Read the model definition and answer for the solid it produces. Units are mm, in the model's axes. A direction names the side the tool comes from. Round coordinates to 2 decimals unless told otherwise and drop trailing zeros. Write each loop counter-clockwise with the first axis right and the second up, starting at its lowest first coordinate (ties: lowest second). Pieces come first, ordered by that corner, then holes. Notation, with made-up numbers: (59.5, -1) -> (112.5, -1) arc R17 ccw to (112.5, 31) -> close; hole circle Ø9 at (67.5, 9). An arc over 180 degrees is marked (long way). Return JSON: item names as keys, results as strings. Group by question number.
(1) The mould has two halves that part along Y. Classify faces 4 (the cylindrical face through (9.127, 29.349, 1.972)), 5 (the cylindrical face through (-0.195, 37.437, 1.972)), 6 (the cylindrical face through (1.014, 38.773, 1.972)): released by +Y, released by -Y, zero draft, split by the parting line, or undercut.
(2) A cutting plane is placed at A-A on y = 25.5. Give the vertices of the cut face in (x, z), then the cut area to 3 significant figures.
(3) Given pin 1 (1.5 mm diameter, centred on x = -10.5, z = 3.5, fed in from -Y); pin 2 (1.5 mm diameter, centred on y = 34.5, z = 1, fed in from +X) (3 decimals), each flat-ended and moving along its own axis, determine where each tip first touches the part or whether it passes through.
(4) Straight lines are drawn through the part: line 1 (Y direction, x = 0, z = 2.2); line 2 (Y direction, x = -15, z = 2); line 3 (X direction, y = 35.75, z = 2.15). For each, find the intervals that lie inside material, in ascending order.
(5) A cutting plane is placed at B-B on z = 3.6. Give the vertices of the cut face in (x, y), then the cut area to 3 significant figures.
(6) A cutting plane is placed at C-C on y = 35.95. Give the vertices of the cut face in (x, z).
(7) For faces 1 (the flat face through (-7, 38.95, 2)), 2 (the flat face through (-11, 20.95, 2)), 3 (the cylindrical face through (5.74, 20.15, 1.97)), determine the directions among +Z, -Z, +X, -X, +Y, -Y from which every point of the face is accessible in a straight line to the end or side of a thin tool.
(8) A cutting plane is placed at D-D on x = -7.5. Give the vertices of the cut face in (y, z).
```python
from build123d import *

# Parameters (mm, degrees)
CROQUIS1_R              = 4
CROQUIS1_R_2            = 2.5
CROQUIS1_R_3            = 1.5
SALIENTE_EXTRUIR1_DEPTH = 4
CORTAR_EXTRUIR1_DEPTH   = 10
REDONDEO1_R             = 10


with BuildPart() as part:
    # Croquis1 → Saliente-Extruir1 (new body)
    with BuildSketch(Plane.XY):
        with BuildLine():
            ThreePointArc((13.175908043, 16.287969402), (20.207859701, 17.03070481), (19.465124293, 24.062656467))
            Line((19.465124293, 24.062656467), (1.886764875, 38.28240612))
            ThreePointArc((1.886764875, 38.28240612), (1.000695169, 38.778181249), (0, 38.95))
            Line((0, 38.95), (-14, 38.95))
            ThreePointArc((-14, 38.95), (-15.75421382, 38.383666755), (-16.84611457, 36.898489248))
            Line((-16.84611457, 36.898489248), (-19.121320344, 30.071320344))
            ThreePointArc((-19.121320344, 30.071320344), (-19.771638598, 29.098050297), (-20, 27.95))
            Line((-20, 27.95), (-20, 23.95))
            ThreePointArc((-20, 23.95), (-19.121320344, 21.828679656), (-17, 20.95))
            Line((-17, 20.95), (-5, 20.95))
            ThreePointArc((-5, 20.95), (-0.298863721, 15.958939945), (4.964272191, 20.353341289))
            ThreePointArc((4.964272191, 20.353341289), (9.295071106, 18.775093958), (13.175908043, 16.287969402))
        make_face()
        with Locations((0, 20.95)):
            Circle(CROQUIS1_R, mode=Mode.SUBTRACT)
        with Locations((-15, 25.95)):
            Circle(CROQUIS1_R_2, mode=Mode.SUBTRACT)
        with Locations((0, 35.95)):
            Circle(CROQUIS1_R_3, mode=Mode.SUBTRACT)
        with Locations((-14, 35.95)):
            Circle(CROQUIS1_R_3, mode=Mode.SUBTRACT)
    extrude(amount=SALIENTE_EXTRUIR1_DEPTH)

    # Croquis2 → Cortar-Extruir1 (cut)
    with BuildSketch(Plane.XY.offset(4)):
        with BuildLine():
            Line((12.087138576, 30.030967124), (6.52630373, 19.907532736))
            ThreePointArc((6.52630373, 19.907532736), (10.015967096, 18.400622357), (13.175908043, 16.287969402))
            ThreePointArc((13.175908043, 16.287969402), (20.207859701, 17.03070481), (19.465124293, 24.062656467))
            Line((19.465124293, 24.062656467), (12.087138576, 30.030967124))
        make_face()
    extrude(amount=-CORTAR_EXTRUIR1_DEPTH, mode=Mode.SUBTRACT)

    # Redondeo1
    redondeo1_edges = [part.edges().sort_by_distance(p)[0] for p in [
        (12.087138576, 30.030967124, 2),
    ]]
    fillet(redondeo1_edges, radius=REDONDEO1_R)


solid = part.part
```
Checks:
{
 "1": {"face 4": "split by the parting line", "face 5": "undercut", "face 6": "released by +Y"},
 "2": {"outline": "(-20, 0) -> (-17.46, 0) -> (-17.46, 4) -> (-20, 4) -> close; (-12.54, 0) -> (9.09, 0) -> (9.09, 4) -> (-12.54, 4) -> close", "area": "96.7 mm^2"},
 "3": {"pin 1": "stops at y = 20.95", "pin 2": "stops at x = 7.115"},
 "4": {"line 1": "y = 15.95 to 16.95, 24.95 to 34.45, 37.45 to 38.95", "line 2": "y = 20.95 to 23.45, 28.45 to 34.83, 37.07 to 38.78", "line 3": "x = -17.23 to -15.49, -12.51 to -1.49, 1.49 to 5.02"},
 "5": {"outline": "(-20, 23.95) arc R3 ccw to (-17, 20.95) -> (-5, 20.95) arc R5 ccw to (4.96, 20.35) arc R20.95 cw to (6.53, 19.91) -> (8.06, 22.7) arc R10 ccw to (5.59, 35.29) -> (1.89, 38.28) arc R3 ccw to (0, 38.95) -> (-14, 38.95) arc R3 ccw to (-16.85, 36.9) -> (-19.12, 30.07) arc R3 ccw to (-20, 27.95) -> close; hole circle Ø5 at (-15, 25.95); hole circle Ø3 at (-14, 35.95); hole circle Ø8 at (0, 20.95); hole circle Ø3 at (0, 35.95)", "area": "424 mm^2"},
 "6": {"outline": "(-17.16, 0) -> (-15.5, 0) -> (-15.5, 4) -> (-17.16, 4) -> close; (-12.5, 0) -> (-1.5, 0) -> (-1.5, 4) -> (-12.5, 4) -> close; (1.5, 0) -> (4.77, 0) -> (4.77, 4) -> (1.5, 4) -> close"},
 "7": {"face 1": "+Z, -Z, +X, -X, +Y", "face 2": "+Z, -Z, -X, -Y", "face 3": "+Z, -Z, -Y"},
 "8": {"outline": "(20.95, 0) -> (38.95, 0) -> (38.95, 4) -> (20.95, 4) -> close"}
}
